from build123d import *

# Parameters (mm, degrees)
F1_DEPTH        = 29
F2_W            = 45.6076951546
F2_H            = 6.2116570825
F3_DEPTH        = 4
F4_W            = 14.4515829202
F4_H            = 20.1
F4_W_2          = 11.8
F5_DEPTH        = 25
F7_D            = 2
F7_DEPTH        = 5
F7_TIP          = 0.600860619
F8_T1_DEPTH     = 29
F8_T3_DEPTH     = 29
F8_T5_DEPTH     = 32.2913124397
F8_T7_DEPTH     = 32.2913124397
F8_T9_DEPTH     = 30.7065545103
F8_T11_DEPTH    = 30.7065545103
F9_R            = 1
F11_D           = 2
F11_DEPTH       = 5
F11_TIP         = 0.600860619
F12_R           = 2
F14_D           = 5.5
F14_CSINK_D     = 11.2
F14_CSINK_ANGLE = 90


# Not quite as in the source:
# - a fillet or chamfer that OpenCascade refuses, or shapes differently, is made with other operations: its cross-section is extruded or revolved along the edge and cut away or added


with BuildPart() as f1:
    # F0 (on Front) → F1 (new body)
    with BuildSketch(Plane.XZ):
        Polygon((45.541646846, 20.7590438725), (-40.0660483086, 20.7590438725), (-52.8151150019, 17.3429417477), (-51.2622007313, 11.54738679), (-40.0660483086, 14.54738679), (45.541646846, 14.54738679), (56.7377992687, 11.54738679), (58.2907135393, 17.3429417477), align=None)
    extrude(amount=F1_DEPTH)

    # F2 (on face) → F3 (join)
    with BuildSketch(Plane.XZ.offset(29)):
        with Locations((2.7377992687, 17.6532153312)):
            Rectangle(F2_W, F2_H)
    extrude(amount=F3_DEPTH)

    # F4 (on face) → F5 (cut)
    with BuildSketch(Plane.XY.offset(20.7590438725)):
        with Locations((-54.240906462, -14.5)):
            Rectangle(F4_W, F4_H)
        with Locations((58.3907135393, -14.5)):
            Rectangle(F4_W_2, F4_H)
    extrude(amount=-F5_DEPTH, mode=Mode.SUBTRACT)

    # F7
    with Locations(Plane(origin=(-47.0151150019, 0, 0), x_dir=(0, -1, 0), z_dir=(-1, 0, 0))):
        with Locations((14.5, 15.7970470638)):
            Hole(F7_D / 2, depth=F7_DEPTH)
            with Locations((0, 0, -(F7_DEPTH + F7_TIP / 2))):  # 118° drill point
                Cone(0, F7_D / 2, F7_TIP, mode=Mode.SUBTRACT)

    # F8: fillet of radius 5 on 6 edges, made by hand

    # F8_s2 → F8_t1 (join)
    with BuildSketch(Plane.XZ):
        with BuildLine():
            ThreePointArc((46.1774795836, 14.3770159214), (45.5360153192, 14.5046110969), (44.8833843581, 14.54738679))
            Line((44.8833843581, 14.54738679), (45.541646846, 14.54738679))
            Line((45.541646846, 14.54738679), (46.1774795836, 14.3770159214))
        make_face()
    extrude(amount=F8_T1_DEPTH)

    # F8_s4 → F8_t3 (join)
    with BuildSketch(Plane.XZ):
        with BuildLine():
            ThreePointArc((-39.4077858206, 14.54738679), (-40.0604167817, 14.5046110969), (-40.7018810462, 14.3770159214))
            Line((-40.7018810462, 14.3770159214), (-40.0660483086, 14.54738679))
            Line((-40.0660483086, 14.54738679), (-39.4077858206, 14.54738679))
        make_face()
    extrude(amount=F8_T3_DEPTH)

    # F8_s6 → F8_t5 (cut)
    with BuildSketch(Plane.XZ.offset(-1.6456562198)):
        with BuildLine():
            ThreePointArc((44.8833843581, 20.7590438725), (45.5360153192, 20.7162681793), (46.1774795836, 20.5886730039))
            Line((46.1774795836, 20.5886730039), (45.541646846, 20.7590438725))
            Line((45.541646846, 20.7590438725), (44.8833843581, 20.7590438725))
        make_face()
    extrude(amount=F8_T5_DEPTH, mode=Mode.SUBTRACT)

    # F8_s8 → F8_t7 (cut)
    with BuildSketch(Plane.XZ.offset(-1.6456562198)):
        with BuildLine():
            ThreePointArc((-39.4077858206, 20.7590438725), (-40.0604167817, 20.7162681793), (-40.7018810462, 20.5886730039))
            Line((-40.7018810462, 20.5886730039), (-40.0660483086, 20.7590438725))
            Line((-40.0660483086, 20.7590438725), (-39.4077858206, 20.7590438725))
        make_face()
    extrude(amount=F8_T7_DEPTH, mode=Mode.SUBTRACT)

    # F8_s10 → F8_t9 (cut)
    with BuildSketch(Plane.XY.offset(2.2999380761)):
        with BuildLine():
            ThreePointArc((20.6426673604, -33), (23.8049450206, -31.8729833462), (25.541646846, -29))
            Line((25.541646846, -29), (25.541646846, -33))
            Line((25.541646846, -33), (20.6426673604, -33))
        make_face()
    extrude(amount=F8_T9_DEPTH, mode=Mode.SUBTRACT)

    # F8_s12 → F8_t11 (cut)
    with BuildSketch(Plane.XY.offset(2.2999380761)):
        with BuildLine():
            ThreePointArc((-20.0660483086, -29), (-18.3293464832, -31.8729833462), (-15.167068823, -33))
            Line((-15.167068823, -33), (-20.0660483086, -33))
            Line((-20.0660483086, -33), (-20.0660483086, -29))
        make_face()
    extrude(amount=F8_T11_DEPTH, mode=Mode.SUBTRACT)

    # F9
    f9_edges = [f1.edges().sort_by_distance(p)[0] for p in [
        (-52.038658, -29, 14.445164),
        (-52.038658, 0, 14.445164),
        (57.514256, 0, 14.445164),
        (57.514256, -29, 14.445164),
    ]]
    fillet(f9_edges, radius=F9_R)

    # F11
    with Locations(Plane.YZ.offset(52.4907135393)):
        with Locations((-14.5, 15.7970470638)):
            Hole(F11_D / 2, depth=F11_DEPTH)
            with Locations((0, 0, -(F11_DEPTH + F11_TIP / 2))):  # 118° drill point
                Cone(0, F11_D / 2, F11_TIP, mode=Mode.SUBTRACT)

    # F12
    f12_edges = [f1.edges().sort_by_distance(p)[0] for p in [
        (-52.038658, -24.55, 14.445164),
        (-52.038658, -4.45, 14.445164),
        (57.514256, -24.55, 14.445164),
        (57.514256, -4.45, 14.445164),
    ]]
    fillet(f12_edges, radius=F12_R)

    # F14 (through all)
    with Locations(Plane.XY.offset(20.7590438725)):
        with Locations((0, -21.3), (0, -8.3)):
            CounterSinkHole(F14_D / 2, F14_CSINK_D / 2, counter_sink_angle=F14_CSINK_ANGLE)


solid = f1.part
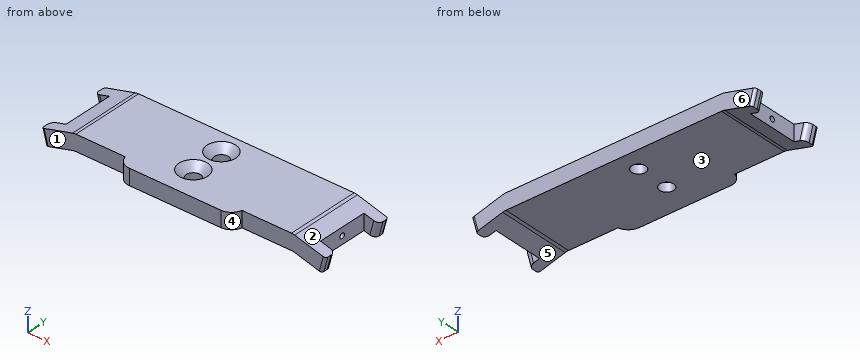
Can you work these out from the model? Positions are in its coordinate system, mm. Face numbers are marked on the shaded views. A direction names the side the tool comes from. Give positions to 0.01 mm unless a question says otherwise; leave off trailing zeros. Write each loop counter-clockwise with the first axis right and the second up, starting at its lowest first coordinate (ties: lowest second). Pieces come first, ordered by that corner, then holes. Notation, with made-up numbers: (-34, 55) -> (22, 55) arc R23 cw to (22, 89) -> close; hole circle Ø1 at (-29, 75). An arc over 180 degrees is marked (long way). Answer as a JSON object with one key per item and string values. Group by question number.
Item 1: Suppose I cut it at B-B (x = 0). Please give me the cut outline in (y, z).
Item 2: I'm going to push flat-ended pins straight in: P1, Ø5, axis at x = 0, y = -8.3, coming from the +Z side; P2, Ø1.2, axis at x = -50, z = 15.5, coming from the -Y side; P3, Ø1.9, axis at y = -17.5, z = 14.5, coming from the +X side; P4, Ø1.6, axis at y = -14.5, z = 15.8, coming from the -X side. Where does each tip first touch, or does it pass through?
Item 3: Please list where these lines run through material, in increasing order: line 1 (Y direction, x = 0, z = 16.4); line 2 (X direction, y = -21.3, z = 16.9); line 3 (Y direction, x = -3, z = 19.25). Write a range as [from, to].
Item 4: For the marked faces 1 and 2, which set-ups out of +Z, -Z, +X, -X, +Y, -Y let a thin tool reach every point of the face, with its end or its side?
Item 5: Suppose I cut it at C-C (x = 49.5). Please give me the cut outline in (y, z), plus the area to 3 significant figures.
Item 6: Suppose I cut it at D-D (x = -37). Please give me the cut outline in (y, z).
Item 7: Suppose I cut it at A-A (y = -8.3). Please give me the cut outline in (x, z).
Item 8: We'd pull the mould along X, two halves only. Please class the marked faces 3, 4, 5 and 6: +X half, -X half, draft (parallel to the pull), parting line (faces both ways), or undercut.
Findings:
{
 "1": {"outline": "(-33, 14.55) -> (-24.05, 14.55) -> (-24.05, 17.91) -> (-26.9, 20.76) -> (-33, 20.76) -> close; (-18.55, 14.55) -> (-11.05, 14.55) -> (-11.05, 17.91) -> (-13.9, 20.76) -> (-15.7, 20.76) -> (-18.55, 17.91) -> close; (-5.55, 14.55) -> (0, 14.55) -> (0, 20.76) -> (-2.7, 20.76) -> (-5.55, 17.91) -> close"},
 "2": {"P1": "passes through", "P2": "stops at y = -29", "P3": "stops at x = 52.49", "P4": "stops at x = -41.9"},
 "3": {"line 1": "y = [-33, -24.05], [-18.55, -11.05], [-5.55, 0]", "line 2": "x = [-47.02, -2.75], [2.75, 52.49]", "line 3": "y = [-33, -24.08], [-18.52, -11.08], [-5.52, 0]"},
 "4": {"face 1": "+Z, -Z, -X, -Y", "face 2": "+Z, +X, +Y, -Y"},
 "5": {"outline": "(-29, 13.49) -> (0, 13.49) -> (0, 19.7) -> (-29, 19.7) -> close; hole circle Ø2 at (-14.5, 15.8)", "area": "177 mm²"},
 "6": {"outline": "(-29, 14.55) -> (0, 14.55) -> (0, 20.76) -> (-29, 20.76) -> close"},
 "7": {"outline": "(-47.02, 12.69) -> (-40.7, 14.38) arc R5 cw to (-39.41, 14.55) -> (-2.75, 14.55) -> (-2.75, 17.91) -> (-5.6, 20.76) -> (-39.41, 20.76) arc R5 ccw to (-40.7, 20.59) -> (-47.02, 18.9) -> close; (2.75, 14.55) -> (44.88, 14.55) arc R5 cw to (46.18, 14.38) -> (52.49, 12.69) -> (52.49, 18.9) -> (46.18, 20.59) arc R5 ccw to (44.88, 20.76) -> (5.6, 20.76) -> (2.75, 17.91) -> close"},
 "8": {"face 3": "undercut", "face 4": "+X half", "face 5": "undercut", "face 6": "draft"}
}
